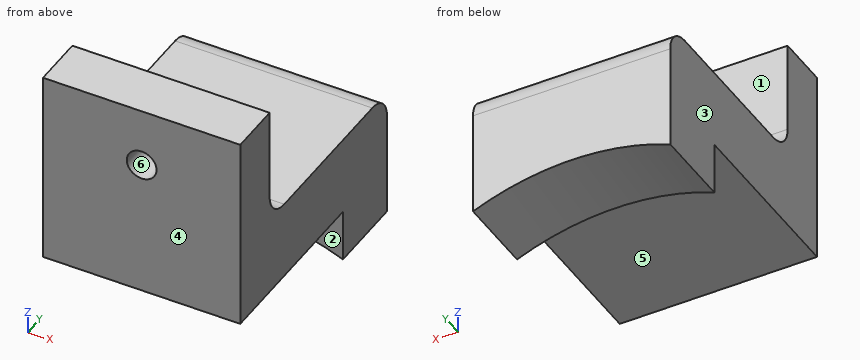
```python
from build123d import *

# Parameters (mm, degrees)
SKETCH1_W                 = 15
SKETCH1_H                 = 10
BOSS_EXTRUDE1_DEPTH       = 6
SKETCH2_R                 = 19.5
CUT_EXTRUDE1_DEPTH        = 9
SKETCH3_W                 = 15
SKETCH3_H                 = 6
BOSS_EXTRUDE2_DEPTH       = 20
SKETCH4_W                 = 15
SKETCH4_H                 = 4
BOSS_EXTRUDE3_DEPTH       = 9
F_4_40_TAPPED_HOLE2_D     = 2.2606
F_4_40_TAPPED_HOLE2_DEPTH = 7.6
F_4_40_TAPPED_HOLE2_TIP   = 0.679152758
FILLET2_R                 = 2


with BuildPart() as part:
    # Sketch1 → Boss-Extrude1 (new body)
    with BuildSketch(Plane(origin=(0, 0, 0), x_dir=(1, 0, 0), z_dir=(0, 1, 0))):
        Rectangle(SKETCH1_W, SKETCH1_H)
    extrude(amount=BOSS_EXTRUDE1_DEPTH)

    # Sketch2 → Cut-Extrude1 (cut)
    with BuildSketch(Plane(origin=(0, 6, 0), x_dir=(1, 0, 0), z_dir=(0, 1, 0))):
        with Locations((0, 23)):
            Circle(SKETCH2_R)
    extrude(amount=-CUT_EXTRUDE1_DEPTH, mode=Mode.SUBTRACT)

    # Sketch3 → Boss-Extrude2 (add)
    with BuildSketch(Plane(origin=(0, 6, 0), x_dir=(1, 0, 0), z_dir=(0, 1, 0))):
        with Locations((0, -2)):
            Rectangle(SKETCH3_W, SKETCH3_H)
    extrude(amount=-BOSS_EXTRUDE2_DEPTH)

    # Sketch4 → Boss-Extrude3 (add)
    with BuildSketch(Plane.XY.offset(5)):
        with Locations((0, -12)):
            Rectangle(SKETCH4_W, SKETCH4_H)
    extrude(amount=BOSS_EXTRUDE3_DEPTH)

    # #4-40 Tapped Hole2
    with Locations(Plane(origin=(0, -14, 0), x_dir=(-1, 0, 0), z_dir=(0, -1, 0))):
        with Locations((0, -9.5)):
            Hole(F_4_40_TAPPED_HOLE2_D / 2, depth=F_4_40_TAPPED_HOLE2_DEPTH)
            with Locations((0, 0, -(F_4_40_TAPPED_HOLE2_DEPTH + F_4_40_TAPPED_HOLE2_TIP / 2))):  # 118° drill point
                Cone(0, F_4_40_TAPPED_HOLE2_D / 2, F_4_40_TAPPED_HOLE2_TIP, mode=Mode.SUBTRACT)

    # Fillet2
    fillet2_edges = [part.edges().sort_by_distance(p)[0] for p in [
        (0, -10, 5),
        (0, 6, 5),
    ]]
    fillet(fillet2_edges, radius=FILLET2_R)


solid = part.part
```
The listing builds one solid part. Answer for the finished solid, in the listing's coordinates (mm). Face numbers are marked on the shaded views. A direction names the side the tool comes from. Round coordinates to 2 decimals unless told otherwise and drop trailing zeros. Loops run counter-clockwise (first coordinate to the right, second up) from the corner with the lowest first, then second, coordinate; pieces in that order, holes last.
Q1. Section D-D, the plane y = -2.75 is taken. Determine the outline of the cut face in (x, z), then the cut area to 3 significant figures.
Q2. Which of the six approach directions +Z, -Z, +X, -X, +Y, -Y give full straight-line access (tool end or side, diameter ignored) to the marked faces 1, 2 and 3?
Q3. Section A-A, the plane z = 9.5 is taken. Determine the outline of the cut face in (x, y), then the cut area to 3 significant figures.
Q4. For a pull along Z with two mould halves and no side action, classify the marked faces 4, 5 and 6 as released by +Z, released by -Z, zero draft, split by the parting line, or undercut.
Q5. Section B-B, the plane x = 0 is taken. Determine the outline of the cut face in (y, z), then the cut area to 3 significant figures.
Q6. Find the intervals of material crossed by line 1 (X direction, y = -12.6, z = 9.5); line 2 (Z direction, x = 0, y = -12); line 3 (Y direction, x = -2.5, z = 9), in increasing order.
Q7. Given pin 1 Ø2 at (x, z) = (3.5, -3) entering from -Y; pin 2 Ø3.5 at (x, z) = (0, 11.5) entering from +Y; pin 3 Ø2 at (x, z) = (0, 9.5) entering from -Y; pin 4 Ø8 at (x, y) = (2, -12) entering from -Z, each flat-ended and moving along its own axis, determine where each tip first touches the part or whether it passes through.
Q8. Section C-C, the plane x = 6.25 is taken. Determine the outline of the cut face in (y, z).
Completed:
1. outline: (-7.5, -1) - (7.5, -1) - (7.5, 5) - (-7.5, 5) - close
1. area: 90.0 mm2
2. face 1: +Z, +X, -X, +Y
2. face 2: -Z, +X, -X, -Y
2. face 3: +Z, -Z, -X, +Y, -Y
3. outline: (-7.5, -14) - (-1.13, -14) - (-1.13, -10) - (-7.5, -10) - close; (1.13, -14) - (7.5, -14) - (7.5, -10) - (1.13, -10) - close
3. area: 51.0 mm2
4. face 4: zero draft
4. face 5: released by -Z
4. face 6: undercut
5. outline: (-14, -1) - (0, -1) - (0, -3.5) - (6, -3.5) - (6, 3) arc R2 ccw to (4, 5) - (-8, 5) arc R2 cw to (-10, 7) - (-10, 8.37) - (-14, 8.37) - close; (-14, 10.63) - (-10, 10.63) - (-10, 14) - (-14, 14) - close
5. area: 162 mm2
6. line 1: x = -7.5 to -1.13, 1.13 to 7.5
6. line 2: z = -1 to 8.37, 10.63 to 14
6. line 3: y = -14 to -10
7. pin 1: stops at y = 0
7. pin 2: stops at y = -10
7. pin 3: passes through
7. pin 4: stops at z = -1
8. outline: (-14, -1) - (0, -1) - (0, -4.53) - (6, -4.53) - (6, 3) arc R2 ccw to (4, 5) - (-8, 5) arc R2 cw to (-10, 7) - (-10, 14) - (-14, 14) - close
